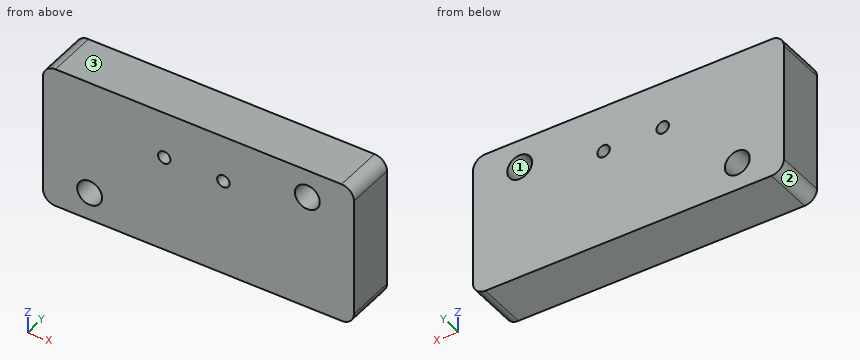
Autodesk Inventor part; units mm, degrees
ref_plane "YZ Plane" through (0, 0, 0) normal (1, 0, 0) x (0, 1, 0)
ref_plane "XZ Plane" through (0, 0, 0) normal (0, 1, 0) x (-1, 0, 0)
ref_plane "XY Plane" through (0, 0, 0) normal (0, 0, 1) x (1, 0, 0)
sketch "Sketch1" plane through (0, 0, 0) normal (0, 1, 0) x (-1, 0, 0)
  line L0 (0, 0) -> (-50, 0)
  line L1 (-50, 0) -> (-50, -23)
  line L2 (-50, -23) -> (0, -23)
  line L3 (0, -23) -> (0, 0)
  dimension "d0" = 50
  dimension "d1" = 23
extrude "Extrusion1" add sketch "Sketch1" along normal blind 8
sketch "Sketch2" plane through (0, 8, 0) normal (0, 1, 0) x (1, 0, 0)
  line L0 (0, 0) -> (50, 0) construction
  line L1 (50, 0) -> (50, 23) construction
  line L2 (50, 23) -> (0, 23) construction
  line L3 (0, 23) -> (0, 0) construction
  point P0 (7.5, 18.5)
  point P1 (19.5, 7.5)
  point P2 (29, 7.5)
  point P3 (42.5, 4.5)
  dimension "d5" = 4.5
  dimension "d6" = 7.5
  dimension "d7" = 7.5
  dimension "d8" = 19.5
  dimension "d9" = 9.5
  dimension "d10" = 7.5
  dimension "d11" = 4.5
hole "Hole1" at (19.5, 8, -7.5) at (29, 8, -7.5) direction (0, -1, 0) diameter 2 end through all
hole "Hole2" at (7.5, 8, -18.5) at (42.5, 8, -4.5) direction (0, -1, 0) diameter 4 end through all
fillet "Fillet1" radius 2 4 edges at (0, 4, 0) (0, 4, -23) (50, 4, 0) (50, 4, -23)
properties part number "A8-0016"
Geometry check sheet. Reference: the model listing, model coordinates, mm. Face numbers are marked on the shaded views. Round coordinates to 2 decimals unless told otherwise and drop trailing zeros. Loops run counter-clockwise (first coordinate to the right, second up) from the corner with the lowest first, then second, coordinate; pieces in that order, holes last.
Item 1: Thickness scan on line 1 (X direction, y = 3, z = -7.5); line 2 (Z direction, x = 29, y = 4.25); line 3 (Z direction, x = 42.5, y = 6.25). Record the ranges inside material, lowest first.
Item 2: Cross-section at C-C on y = 1.5. Record the boundary of the cut face in (x, z).
Item 3: Cross-section at B-B on z = -7.5. Record the boundary of the cut face in (x, y), then the cut area to 3 significant figures.
Item 4: Cross-section at D-D on z = -4.5. Record the boundary of the cut face in (x, y), then the cut area to 3 significant figures.
Item 5: Cross-section at A-A on x = 19.5. Record the boundary of the cut face in (y, z), then the cut area to 3 significant figures.
Item 6: Gauge pin test, flat end, axial feed: pin 1 (3 mm diameter, centred on x = 42.5, z = -4.5, fed in from -Y). Record the tip position at first contact, or that the pin passes through.
Item 7: Mould release check, pull along X, two halves, no side actions. Record for the marked faces 1, 2 and 3: pulls with the +X half, pulls with the -X half, needs draft (parallel to the pull), parting line crosses it, or undercut.
Answer sheet:
1. line 1: x = 0 to 18.5, 20.5 to 28, 30 to 50
1. line 2: z = -23 to -8.5, -6.5 to 0
1. line 3: z = -23 to -6.5, -2.5 to 0
2. outline: (0, -21) arc R2 ccw to (2, -23) - (48, -23) arc R2 ccw to (50, -21) - (50, -2) arc R2 ccw to (48, 0) - (2, 0) arc R2 ccw to (0, -2) - close; hole circle Ø4 at (7.5, -18.5); hole circle Ø2 at (19.5, -7.5); hole circle Ø2 at (29, -7.5); hole circle Ø4 at (42.5, -4.5)
3. outline: (0, 0) - (18.5, 0) - (18.5, 8) - (0, 8) - close; (20.5, 0) - (28, 0) - (28, 8) - (20.5, 8) - close; (30, 0) - (50, 0) - (50, 8) - (30, 8) - close
3. area: 368 mm2
4. outline: (0, 0) - (40.5, 0) - (40.5, 8) - (0, 8) - close; (44.5, 0) - (50, 0) - (50, 8) - (44.5, 8) - close
4. area: 368 mm2
5. outline: (0, -23) - (8, -23) - (8, -8.5) - (0, -8.5) - close; (0, -6.5) - (8, -6.5) - (8, 0) - (0, 0) - close
5. area: 168 mm2
6. pin 1: passes through
7. face 1: undercut
7. face 2: pulls with the -X half
7. face 3: needs draft
